Source: CAD feature listing. Evaluate the final solid. Frame: model axes, mm. A direction names the side the tool comes from. Coordinates: 2 decimals unless noted, no trailing zeros. Write each loop counter-clockwise with the first axis right and the second up, starting at its lowest first coordinate (ties: lowest second). Pieces come first, ordered by that corner, then holes. Notation, with made-up numbers: (45.25, 2.5) -> (68.25, 2.5) arc R19 cw to (68.25, 21.5) -> close; hole circle Ø2 at (17.25, 39). An arc over 180 degrees is marked (long way). Write item = value, one per line.
from build123d import *

# Parameters (mm, degrees)
SKETCH_R  = 1.8288
PAD_DEPTH = 3


with BuildPart() as part:
    # Sketch → Pad (new body)
    with BuildSketch(Plane.XY):
        with BuildLine():
            ThreePointArc((-75.2, 50.8), (-75.907107, 50.507107), (-76.2, 49.8))
            Line((-76.2, -49.8), (-76.2, 49.8))
            ThreePointArc((-76.2, -49.8), (-75.907107, -50.507107), (-75.2, -50.8))
            Line((-75.2, -50.8), (-61.452, -50.8))
            ThreePointArc((-61.452, -50.8), (-60.744893, -50.507107), (-60.452, -49.8))
            Line((-60.452, -38.1), (-60.452, -49.8))
            ThreePointArc((-53.848, -38.1), (-57.15, -34.797985), (-60.452, -38.1))
            Line((-53.848, -38.1), (-53.848, -49.8))
            ThreePointArc((-53.848, -49.8), (-53.555107, -50.507107), (-52.848, -50.8))
            Line((-52.848, -50.8), (2.048, -50.8))
            ThreePointArc((2.048, -50.8), (2.755107, -50.507107), (3.048, -49.8))
            Line((3.048, -38.1), (3.048, -49.8))
            ThreePointArc((9.652, -38.1), (6.35, -34.797989), (3.048, -38.1))
            Line((9.652, -38.1), (9.652, -49.8))
            ThreePointArc((9.652, -49.8), (9.944893, -50.507107), (10.652, -50.8))
            Line((10.652, -50.8), (75.2, -50.8))
            ThreePointArc((75.2, -50.8), (75.907107, -50.507107), (76.2, -49.8))
            Line((76.2, 49.8), (76.2, -49.8))
            ThreePointArc((76.2, 49.8), (75.907107, 50.507107), (75.2, 50.8))
            Line((-75.2, 50.8), (75.2, 50.8))
        make_face()
        with Locations((-65.7352, 44.45)):
            Circle(SKETCH_R, mode=Mode.SUBTRACT)
        with Locations((65.7352, 44.45)):
            Circle(SKETCH_R, mode=Mode.SUBTRACT)
    extrude(amount=PAD_DEPTH)


solid = part.part
1) Material intervals for probe 1 along X at (y, z) = (-43, 1.1); probe 2 along Y at (x, z) = (66, 1.4); probe 3 along Y at (x, z) = (-64.5, 0.95), sorted ascending. Write a range as [from, to].
Answer block:
probe_1 = [-76.2, -60.45], [-53.85, 3.05], [9.65, 76.2]
probe_2 = [-50.8, 42.64], [46.26, 50.8]
probe_3 = [-50.8, 43.1], [45.8, 50.8]
2) Reachability of faces 1 (the flat face through (-68, -50.8, 1)), 2 (the flat face through (3.048, -44, 1)) from +Z, -Z, +X, -X, +Y, -Y: full face, straight path, thin tool, end or side. Return the list, or none.
Answer block:
face_1 = +Z, -Z, +X, -X, -Y
face_2 = +Z, -Z, -Y
3) Cut plane A-A, the plane y = 44.45. Output: boundary loops of the cut face in (x, z).
Answer block:
outline = (-76.2, 0) -> (-67.56, 0) -> (-67.56, 3) -> (-76.2, 3) -> close; (-63.91, 0) -> (63.91, 0) -> (63.91, 3) -> (-63.91, 3) -> close; (67.56, 0) -> (76.2, 0) -> (76.2, 3) -> (67.56, 3) -> close
4) First-contact query: pin 1 Ø4 at (x, y) = (61, 3) entering from -Z. Flat tip, straight axial feed; report the tip coordinate or a pass-through.
Answer block:
pin_1 = 0
5) Cut plane B-B, the plane x = 6.35. Output: boundary loops of the cut face in (y, z).
Answer block:
outline = (-34.8, 0) -> (50.8, 0) -> (50.8, 3) -> (-34.8, 3) -> close
